```python
from build123d import *

# Parameters (mm, degrees)
SKETCH1_W               = 10
SKETCH1_H               = 7.6
EXTRUDE1_DEPTH          = 10
SKETCH2_OUTSIDE_W       = 12.81
SKETCH2_OUTSIDE_H       = 15.21
CUT_EXTRUDE1_DEPTH      = 6
CUT_EXTRUDE1_DEPTH_BACK = 6
SKETCH3_R               = 1.65
SKETCH3_R_2             = 0.35
SKETCH3_W               = 0.4
SKETCH3_H               = 4
CUT_EXTRUDE2_DEPTH      = 4
SKETCH4_W               = 4
SKETCH4_H               = 5.5
CUT_EXTRUDE3_DEPTH      = 5.6
SKETCH5_W               = 4
SKETCH5_H               = 5.1
EXTRUDE2_DEPTH          = 4.25
SKETCH6_R               = 1.6
CUT_EXTRUDE4_DEPTH      = 4.25
EXTRUDE3_DEPTH          = 6.5
CUT_EXTRUDE5_DEPTH      = 6.5
SKETCH10_W              = 1.1
SKETCH10_H              = 0.5
CUT_EXTRUDE6_DEPTH      = 3.6
SKETCH11_R              = 0.5
EXTRUDE4_DEPTH          = 3.5
SKETCH12_R              = 1.65
EXTRUDE5_DEPTH          = 3
CUT_EXTRUDE7_DEPTH      = 0.4
EXTRUDE6_DEPTH          = 0.945
EXTRUDE9_DEPTH          = 0.39
LPATTERN1_COUNT         = 2
LPATTERN1_PITCH         = 5
FILLET1_R               = 0.3
FILLET2_R               = 0.7
SCALE1_SCALE            = 0.7


with BuildPart() as part:
    # Sketch1 → Extrude1 (new body)
    with BuildSketch(Plane(origin=(0, 0, 0), x_dir=(1, 0, 0), z_dir=(0, 1, 0))):
        Rectangle(SKETCH1_W, SKETCH1_H)
    extrude(amount=EXTRUDE1_DEPTH)

    # Sketch2 outside → Cut-Extrude1 (cut, two sides)
    with BuildSketch(Plane(origin=(0, 0, 0), x_dir=(0, 0, -1), z_dir=(1, 0, 0))) as cut_extrude1_sk:
        with Locations((0, 5)):
            Rectangle(SKETCH2_OUTSIDE_W, SKETCH2_OUTSIDE_H)
        Polygon((2.5, 10), (3.8, 6.5), (3.8, 0), (-3.8, 0), (-3.8, 6.5), (-2.5, 10), align=None, mode=Mode.SUBTRACT)
    extrude(amount=CUT_EXTRUDE1_DEPTH, mode=Mode.SUBTRACT)
    extrude(cut_extrude1_sk.sketch, amount=-CUT_EXTRUDE1_DEPTH_BACK, mode=Mode.SUBTRACT)

    # Sketch3 → Cut-Extrude2 (cut)
    with BuildSketch(Plane(origin=(0, 10, 0), x_dir=(-1, 0, 0), z_dir=(0, 1, 0))):
        with Locations((2.5, 0)):
            Circle(SKETCH3_R)
        with Locations((-2.5, 0)):
            Circle(SKETCH3_R)
        with Locations((2.5, -2.78)):
            Circle(SKETCH3_R_2)
        with Locations((-2.5, -2.78)):
            Circle(SKETCH3_R_2)
        Rectangle(SKETCH3_W, SKETCH3_H)
    extrude(amount=-CUT_EXTRUDE2_DEPTH, mode=Mode.SUBTRACT)

    # Sketch4 → Cut-Extrude3 (cut)
    with BuildSketch(Plane.XY.offset(3.8)):
        with Locations((-2.5, 3.25)):
            Rectangle(SKETCH4_W, SKETCH4_H)
        with Locations((2.5, 3.25)):
            Rectangle(SKETCH4_W, SKETCH4_H)
    extrude(amount=-CUT_EXTRUDE3_DEPTH, mode=Mode.SUBTRACT)

    # Sketch5 → Extrude2 (add)
    with BuildSketch(Plane.XY.offset(-1.8)):
        with Locations((-2.5, 3.05)):
            Rectangle(SKETCH5_W, SKETCH5_H)
        with Locations((2.5, 3.05)):
            Rectangle(SKETCH5_W, SKETCH5_H)
    extrude(amount=EXTRUDE2_DEPTH)

    # Sketch6 → Cut-Extrude4 (cut)
    with BuildSketch(Plane.XY.offset(2.45)):
        with Locations((-2.5, 2.554263468)):
            Circle(SKETCH6_R)
        with Locations((2.5, 2.554263468)):
            Circle(SKETCH6_R)
    extrude(amount=-CUT_EXTRUDE4_DEPTH, mode=Mode.SUBTRACT)

    # Sketch7 → Extrude3 (add)
    with BuildSketch(Plane(origin=(0, 0, 0), x_dir=(1, 0, 0), z_dir=(0, 1, 0))):
        Polygon((-5.6, 3.1), (-5, 2.881617859), (-5, 2.118382141), (-5.6, 1.9), align=None)
    extrude(amount=EXTRUDE3_DEPTH)

    # Sketch9 → Cut-Extrude5 (cut)
    with BuildSketch(Plane(origin=(0, 0, 0), x_dir=(1, 0, 0), z_dir=(0, 1, 0))):
        Polygon((5, 2.881617859), (4.4, 3.1), (4.4, 1.9), (5, 2.118382141), align=None)
    extrude(amount=CUT_EXTRUDE5_DEPTH, mode=Mode.SUBTRACT)

    # Sketch10 → Cut-Extrude6 (cut)
    with BuildSketch(Plane.XY.offset(3.8)):
        with Locations((-2.5, 0.25)):
            Rectangle(SKETCH10_W, SKETCH10_H)
        with Locations((2.5, 0.25)):
            Rectangle(SKETCH10_W, SKETCH10_H)
    extrude(amount=-CUT_EXTRUDE6_DEPTH, mode=Mode.SUBTRACT)

    # Sketch11 → Extrude4 (add)
    with BuildSketch(Plane.XZ.offset(-0.5)):
        with Locations((-2.5, 0.8)):
            Circle(SKETCH11_R)
        with Locations((2.5, 0.8)):
            Circle(SKETCH11_R)
    extrude(amount=EXTRUDE4_DEPTH)

    # Sketch12 → Extrude5 (add)
    with BuildSketch(Plane.XZ.offset(-6)):
        with Locations((2.5, 0)):
            Circle(SKETCH12_R)
        with Locations((-2.5, 0)):
            Circle(SKETCH12_R)
    extrude(amount=-EXTRUDE5_DEPTH)

    # Sketch13 → Cut-Extrude7 (cut)
    with BuildSketch(Plane(origin=(0, 9, 0), x_dir=(-1, 0, 0), z_dir=(0, 1, 0))):
        with BuildLine():
            Line((3.594307251, -1.234905519), (1.825829895, 1.505986278))
            ThreePointArc((1.825829895, 1.505986278), (1.605433494, 1.386452583), (1.405692749, 1.234905519))
            Line((1.405692749, 1.234905519), (3.174170105, -1.505986278))
            ThreePointArc((3.174170105, -1.505986278), (3.394566506, -1.386452583), (3.594307251, -1.234905519))
        make_face()
        with BuildLine():
            Line((-2.83217089, -1.616218581), (-1.698971441, 1.44251629))
            ThreePointArc((-1.698971441, 1.44251629), (-1.926782442, 1.54723031), (-2.16782911, 1.616218581))
            Line((-2.16782911, 1.616218581), (-3.301028559, -1.44251629))
            ThreePointArc((-3.301028559, -1.44251629), (-3.073217558, -1.54723031), (-2.83217089, -1.616218581))
        make_face()
    extrude(amount=-CUT_EXTRUDE7_DEPTH, mode=Mode.SUBTRACT)

    # Sketch14 → Extrude6 (add, symmetric)
    with BuildSketch(Plane.ZY.offset(2.5)):
        Polygon((2.45, 5.6), (3.03887637, 3.861674443), (0.167170254, 1.787608865), (-0.546359637, 2.097431054), (-0.705673534, 1.730526322), (0.216750724, 1.33), (3.512480259, 3.710312924), (2.736824279, 6), (-1.8, 6), (-1.8, 5.6), align=None)
    extrude6 = extrude(amount=EXTRUDE6_DEPTH, both=True)

    # Sketch15 → Extrude9 (add)
    with BuildSketch(Plane(origin=(0, 1.449355072, 4.278403908), x_dir=(1, 0, 0), z_dir=(0, 0.320850379, 0.947129893))):
        Polygon((-1.555, 4.8), (-1.555, 2.903968921), (-0.51, 4.8), align=None)
        Polygon((-3.445, 4.8), (-3.445, 2.903968921), (-4.49, 4.8), align=None)
    extrude9 = extrude(amount=-EXTRUDE9_DEPTH)

    # LPattern1: Extrude6, Extrude9 ×2
    with Locations(*[(i * LPATTERN1_PITCH, 0, 0) for i in range(1, LPATTERN1_COUNT)]):
        add(extrude6)
        add(extrude9)

    # Fillet1
    fillet1_edges = [part.edges().sort_by_distance(p)[0] for p in [
        (-2.5, 3.861674443, 3.03887637),
        (-2.5, 1.787608865, 0.167170254),
        (2.5, 3.861674443, 3.03887637),
        (2.5, 1.787608865, 0.167170254),
    ]]
    fillet(fillet1_edges, radius=FILLET1_R)

    # Fillet2
    fillet2_edges = [part.edges().sort_by_distance(p)[0] for p in [
        (-2.5, 3.710312924, 3.512480259),
        (-2.5, 1.33, 0.216750724),
        (2.5, 1.33, 0.216750724),
        (2.5, 3.710312924, 3.512480259),
    ]]
    fillet(fillet2_edges, radius=FILLET2_R)


with BuildPart() as part_1:
    # Scale1: scaled about (0, 0, 0)
    add(part.part.scale(SCALE1_SCALE))


solid = part_1.part
```
The listing builds one solid part. Answer for the finished solid, in the listing's coordinates (mm). A direction names the side the tool comes from. Coordinates: 2 decimals unless noted, no trailing zeros. Loops run counter-clockwise (first coordinate to the right, second up) from the corner with the lowest first, then second, coordinate; pieces in that order, holes last. Notation, with made-up numbers: (-31, 81) - (-6, 81) arc R15 cw to (-6, 85) - close; hole circle Ø2 at (23.25, 63). An arc over 180 degrees is marked (long way). Use a Markdown table: item, result. Add a question column.
1) For faces 3 (the flat face through (-1, 0.35, 2)), 4 (the flat face through (0, 2, 2.66)), 5 (the flat face through (-1.759, 1.976, 1.12)), 6 (the flat face through (2.4, 6.3, 0.3)), determine the directions among +Z, -Z, +X, -X, +Y, -Y from which every point of the face is accessible in a straight line to the end or side of a thin tool.
2) The part is cut by section A-A, the plane y = -1. Give the vertices of the cut face in (x, z), and give its area (3 significant figures).
3) The mould has two halves that part along X. Classify faces 1 (the flat face through (0.05, 5.79, -2.2)), 2 (the flat face through (0.8, 4.2, 1.2)): released by +X, released by -X, zero draft, split by the parting line, or undercut.
4) The part is cut by section B-B, the plane z = 0.56. State how many separate pieces and enclosed holes the cut face has, and give its area (3 significant figures).
5) Given pin 1 (3 mm diameter, centred on x = 2, z = 0.5, fed in from +Y); pin 2 (1.2 mm diameter, centred on x = -2, z = 0, fed in from +Y), each flat-ended and moving along its own axis, determine where each tip first touches the part or whether it passes through.
6) Find the intervals of material crossed by line 1 (X direction, y = 2.5, z = 2.1); line 2 (X direction, y = 1.5, z = -0.9); line 3 (Z direction, x = -1.75, y = 6.55) (3 decimals), in increasing order.
7) The part is cut by section C-C, the plane y = 5.75. Give the vertices of the cut face in (x, z) (3 decimals), and give its area (3 significant figures).
Here are the results:
| question | item | result |
|---|---|---|
| 1 | face 3 | +Z |
| 1 | face 4 | +Z, +X, -X, +Y, -Y |
| 1 | face 5 | none |
| 1 | face 6 | +Y |
| 2 | outline | circle Ø0.7 at (-1.75, 0.56); circle Ø0.7 at (1.75, 0.56) |
| 2 | area | 0.770 mm^2 |
| 3 | face 1 | zero draft |
| 3 | face 2 | undercut |
| 4 | separate pieces | 3 |
| 4 | enclosed holes | 6 |
| 4 | area | 40.3 mm^2 |
| 5 | pin 1 | stops at y = 7 |
| 5 | pin 2 | stops at y = 6.3 |
| 6 | line 1 | x = -3.5 to -3.15, -2.41 to -1.09, -0.35 to 0.35, 1.09 to 2.41, 3.15 to 3.5 |
| 6 | line 2 | x = -3.5 to -2.83, -0.67 to 0.67, 2.83 to 3.5 |
| 6 | line 3 | z = -1.701 to -1.155, 1.155 to 1.917 |
| 7 | outline | (-3.5, -2.214) - (3.5, -2.214) - (3.5, 2.214) - (-3.5, 2.214) - close; hole circle Ø0.49 at (-1.75, -1.946); hole (-0.14, -1.4) - (0.14, -1.4) - (0.14, 1.4) - (-0.14, 1.4) - close; hole circle Ø0.49 at (1.75, -1.946) |
| 7 | area | 29.8 mm^2 |
